from build123d import *

# Parameters (mm, degrees)
SKETCH1_W                  = 323
SKETCH1_H                  = 236
SKETCH1_W_2                = 286.7
SKETCH1_H_2                = 199.7
BOSS_EXTRUDE1_DEPTH        = 5
SKETCH2_W                  = 323
SKETCH2_H                  = 236
SKETCH2_W_2                = 297.2
SKETCH2_H_2                = 210.2
BOSS_EXTRUDE2_DEPTH        = 3.2
FILLET1_R                  = 10
FILLET2_R                  = 20
M4_TAPPED_HOLE1_AT_2_COUNT = 2
M4_TAPPED_HOLE1_AT_2_PITCH = 66.8
M4_TAPPED_HOLE1_AT_3_COUNT = 2
M4_TAPPED_HOLE1_AT_3_PITCH = 133.6
M4_TAPPED_HOLE1_AT_4_COUNT = 2
M4_TAPPED_HOLE1_AT_4_PITCH = 200.4
M4_TAPPED_HOLE1_AT_5_COUNT = 2
M4_TAPPED_HOLE1_AT_5_PITCH = 267.2
M4_TAPPED_HOLE2_AT_2_COUNT = 2
M4_TAPPED_HOLE2_AT_2_PITCH = 45.05
M4_TAPPED_HOLE2_AT_3_COUNT = 2
M4_TAPPED_HOLE2_AT_3_PITCH = 90.1
M4_TAPPED_HOLE2_AT_4_COUNT = 2
M4_TAPPED_HOLE2_AT_4_PITCH = 135.15
M4_TAPPED_HOLE2_AT_5_COUNT = 2
M4_TAPPED_HOLE2_AT_5_PITCH = 180.2
CHAMFER2_SIZE              = 3
SKETCH7_R                  = 3
CUT_EXTRUDE1_DEPTH         = 3.2
FILLET3_R                  = 10
CHAMFER3_SIZE              = 1
CUT_EXTRUDE2_DEPTH         = 2
CUT_EXTRUDE3_DEPTH         = 2


with BuildPart() as part:
    # Sketch1 → Boss-Extrude1 (new body)
    with BuildSketch(Plane(origin=(0, 0, 0), x_dir=(1, 0, 0), z_dir=(0, 1, 0))):
        Rectangle(SKETCH1_W, SKETCH1_H)
        Rectangle(SKETCH1_W_2, SKETCH1_H_2, mode=Mode.SUBTRACT)
    extrude(amount=BOSS_EXTRUDE1_DEPTH)

    # Sketch2 → Boss-Extrude2 (add)
    with BuildSketch(Plane.XZ):
        Rectangle(SKETCH2_W, SKETCH2_H)
        Rectangle(SKETCH2_W_2, SKETCH2_H_2, mode=Mode.SUBTRACT)
    extrude(amount=BOSS_EXTRUDE2_DEPTH)

    # Fillet1
    fillet1_edges = [part.edges().sort_by_distance(p)[0] for p in [
        (-143.35, 2.5, 99.85),
        (143.35, 2.5, 99.85),
        (143.35, 2.5, -99.85),
        (-143.35, 2.5, -99.85),
    ]]
    fillet(fillet1_edges, radius=FILLET1_R)

    # Fillet2
    fillet2_edges = [part.edges().sort_by_distance(p)[0] for p in [
        (-161.5, 0.9, 118),
        (-161.5, 0.9, -118),
        (161.5, 0.9, -118),
        (161.5, 0.9, 118),
    ]]
    fillet(fillet2_edges, radius=FILLET2_R)

    # Sketch4 → M4 Tapped Hole1 (revolve, cut)
    with BuildSketch(Plane(origin=(133.6, -3.2, -109), x_dir=(0, 0, -1), z_dir=(1, 0, 0))):
        Polygon((0, 0), (0, 6.991420021), (1.65, 6), (1.65, 0), align=None)
    m4_tapped_hole1 = revolve(axis=Axis((133.6, -9.55, -109), (0, 1, 0)), mode=Mode.SUBTRACT)

    # M4 Tapped Hole1 at 2: M4 Tapped Hole1 ×2
    with Locations(*[(-i * M4_TAPPED_HOLE1_AT_2_PITCH, 0, 0) for i in range(1, M4_TAPPED_HOLE1_AT_2_COUNT)]):
        add(m4_tapped_hole1, mode=Mode.SUBTRACT)

    # M4 Tapped Hole1 at 3: M4 Tapped Hole1 ×2
    with Locations(*[(-i * M4_TAPPED_HOLE1_AT_3_PITCH, 0, 0) for i in range(1, M4_TAPPED_HOLE1_AT_3_COUNT)]):
        add(m4_tapped_hole1, mode=Mode.SUBTRACT)

    # M4 Tapped Hole1 at 4: M4 Tapped Hole1 ×2
    with Locations(*[(-i * M4_TAPPED_HOLE1_AT_4_PITCH, 0, 0) for i in range(1, M4_TAPPED_HOLE1_AT_4_COUNT)]):
        add(m4_tapped_hole1, mode=Mode.SUBTRACT)

    # M4 Tapped Hole1 at 5: M4 Tapped Hole1 ×2
    with Locations(*[(-i * M4_TAPPED_HOLE1_AT_5_PITCH, 0, 0) for i in range(1, M4_TAPPED_HOLE1_AT_5_COUNT)]):
        add(m4_tapped_hole1, mode=Mode.SUBTRACT)

    # Mirror1: M4 Tapped Hole1 across plane
    add(m4_tapped_hole1.mirror(Plane.XY), mode=Mode.SUBTRACT)

    # Mirror1 copy 1 sketch → Mirror1 copy 1 (revolve, cut)
    with BuildSketch(Plane(origin=(66.8, -3.2, 109), x_dir=(0, 0, 1), z_dir=(1, 0, 0))):
        Polygon((0, 0), (0, -6.991420021), (1.65, -6), (1.65, 0), align=None)
    revolve(axis=Axis((66.8, -9.55, 109), (0, -1, 0)), mode=Mode.SUBTRACT)

    # Mirror1 copy 2 sketch → Mirror1 copy 2 (revolve, cut)
    with BuildSketch(Plane(origin=(0, -3.2, 109), x_dir=(0, 0, 1), z_dir=(1, 0, 0))):
        Polygon((0, 0), (0, -6.991420021), (1.65, -6), (1.65, 0), align=None)
    revolve(axis=Axis((0, -9.55, 109), (0, -1, 0)), mode=Mode.SUBTRACT)

    # Mirror1 copy 3 sketch → Mirror1 copy 3 (revolve, cut)
    with BuildSketch(Plane(origin=(-66.8, -3.2, 109), x_dir=(0, 0, 1), z_dir=(1, 0, 0))):
        Polygon((0, 0), (0, -6.991420021), (1.65, -6), (1.65, 0), align=None)
    revolve(axis=Axis((-66.8, -9.55, 109), (0, -1, 0)), mode=Mode.SUBTRACT)

    # Mirror1 copy 4 sketch → Mirror1 copy 4 (revolve, cut)
    with BuildSketch(Plane(origin=(-133.6, -3.2, 109), x_dir=(0, 0, 1), z_dir=(1, 0, 0))):
        Polygon((0, 0), (0, -6.991420021), (1.65, -6), (1.65, 0), align=None)
    revolve(axis=Axis((-133.6, -9.55, 109), (0, -1, 0)), mode=Mode.SUBTRACT)

    # Sketch6 → M4 Tapped Hole2 (revolve, cut)
    with BuildSketch(Plane(origin=(152.5, -3.2, -90.1), x_dir=(0, 0, -1), z_dir=(1, 0, 0))):
        Polygon((0, 0), (0, 7.091420021), (1.65, 6.1), (1.65, 0), align=None)
    m4_tapped_hole2 = revolve(axis=Axis((152.5, -9.55, -90.1), (0, 1, 0)), mode=Mode.SUBTRACT)

    # M4 Tapped Hole2 at 2: M4 Tapped Hole2 ×2
    with Locations(*[(0, 0, i * M4_TAPPED_HOLE2_AT_2_PITCH) for i in range(1, M4_TAPPED_HOLE2_AT_2_COUNT)]):
        add(m4_tapped_hole2, mode=Mode.SUBTRACT)

    # M4 Tapped Hole2 at 3: M4 Tapped Hole2 ×2
    with Locations(*[(0, 0, i * M4_TAPPED_HOLE2_AT_3_PITCH) for i in range(1, M4_TAPPED_HOLE2_AT_3_COUNT)]):
        add(m4_tapped_hole2, mode=Mode.SUBTRACT)

    # M4 Tapped Hole2 at 4: M4 Tapped Hole2 ×2
    with Locations(*[(0, 0, i * M4_TAPPED_HOLE2_AT_4_PITCH) for i in range(1, M4_TAPPED_HOLE2_AT_4_COUNT)]):
        add(m4_tapped_hole2, mode=Mode.SUBTRACT)

    # M4 Tapped Hole2 at 5: M4 Tapped Hole2 ×2
    with Locations(*[(0, 0, i * M4_TAPPED_HOLE2_AT_5_PITCH) for i in range(1, M4_TAPPED_HOLE2_AT_5_COUNT)]):
        add(m4_tapped_hole2, mode=Mode.SUBTRACT)

    # Mirror2: M4 Tapped Hole2 across plane
    add(m4_tapped_hole2.mirror(Plane(origin=(0, 0, 0), x_dir=(0, 0, 1), z_dir=(1, 0, 0))), mode=Mode.SUBTRACT)

    # Mirror2 copy 1 sketch → Mirror2 copy 1 (revolve, cut)
    with BuildSketch(Plane(origin=(-152.5, -3.2, -45.05), x_dir=(0, 0, -1), z_dir=(-1, 0, 0))):
        Polygon((0, 0), (0, -7.091420021), (1.65, -6.1), (1.65, 0), align=None)
    revolve(axis=Axis((-152.5, -9.55, -45.05), (0, -1, 0)), mode=Mode.SUBTRACT)

    # Mirror2 copy 2 sketch → Mirror2 copy 2 (revolve, cut)
    with BuildSketch(Plane(origin=(-152.5, -3.2, 0), x_dir=(0, 0, -1), z_dir=(-1, 0, 0))):
        Polygon((0, 0), (0, -7.091420021), (1.65, -6.1), (1.65, 0), align=None)
    revolve(axis=Axis((-152.5, -9.55, 0), (0, -1, 0)), mode=Mode.SUBTRACT)

    # Mirror2 copy 3 sketch → Mirror2 copy 3 (revolve, cut)
    with BuildSketch(Plane(origin=(-152.5, -3.2, 45.05), x_dir=(0, 0, -1), z_dir=(-1, 0, 0))):
        Polygon((0, 0), (0, -7.091420021), (1.65, -6.1), (1.65, 0), align=None)
    revolve(axis=Axis((-152.5, -9.55, 45.05), (0, -1, 0)), mode=Mode.SUBTRACT)

    # Mirror2 copy 4 sketch → Mirror2 copy 4 (revolve, cut)
    with BuildSketch(Plane(origin=(-152.5, -3.2, 90.1), x_dir=(0, 0, -1), z_dir=(-1, 0, 0))):
        Polygon((0, 0), (0, -7.091420021), (1.65, -6.1), (1.65, 0), align=None)
    revolve(axis=Axis((-152.5, -9.55, 90.1), (0, -1, 0)), mode=Mode.SUBTRACT)

    # Chamfer2
    chamfer2_edges = [part.edges().sort_by_distance(p)[0] for p in [
        (0, 5, 118),
        (-161.5, 5, 0),
        (161.5, 5, 0),
        (0, 5, -118),
        (-155.642135624, 5, -112.142135624),
        (155.642135624, 5, 112.142135624),
        (155.642135624, 5, -112.142135624),
        (-155.642135624, 5, 112.142135624),
    ]]
    chamfer(chamfer2_edges, length=CHAMFER2_SIZE)

    # Sketch7 → Cut-Extrude1 (cut)
    with BuildSketch(Plane.XZ.offset(3.2)):
        with Locations((147.3, -103.8)):
            Circle(SKETCH7_R)
        with Locations((-147.3, -103.8)):
            Circle(SKETCH7_R)
        with Locations((-147.3, 103.8)):
            Circle(SKETCH7_R)
        with Locations((147.3, 103.8)):
            Circle(SKETCH7_R)
    extrude(amount=-CUT_EXTRUDE1_DEPTH, mode=Mode.SUBTRACT)

    # Fillet3
    fillet3_edges = [part.edges().sort_by_distance(p)[0] for p in [
        (144.596298833, -1.6, -105.1),
        (-144.596298833, -1.6, -105.1),
        (-148.6, -1.6, 101.096298833),
        (144.596298833, -1.6, 105.1),
        (148.6, -1.6, 101.096298833),
        (-144.596298833, -1.6, 105.1),
        (-148.6, -1.6, -101.096298833),
        (148.6, -1.6, -101.096298833),
    ]]
    fillet(fillet3_edges, radius=FILLET3_R)

    # Chamfer3
    chamfer3_edges = [part.edges().sort_by_distance(p)[0] for p in [
        (0, 5, 99.85),
        (143.35, 5, 0),
        (0, 5, -99.85),
        (-143.35, 5, 0),
        (140.421067812, 5, 96.921067812),
        (140.421067812, 5, -96.921067812),
        (-140.421067812, 5, 96.921067812),
        (-140.421067812, 5, -96.921067812),
    ]]
    chamfer(chamfer3_edges, length=CHAMFER3_SIZE)

    # Sketch8 → Cut-Extrude2 (cut)
    with BuildSketch(Plane.XZ):
        with BuildLine():
            Line((148.6, -89.85), (148.6, 89.85))
            ThreePointArc((148.6, 89.85), (144.133378413, 100.633378413), (133.35, 105.1))
            Line((133.35, 105.1), (-133.35, 105.1))
            ThreePointArc((-133.35, 105.1), (-144.133378413, 100.633378413), (-148.6, 89.85))
            Line((-148.6, 89.85), (-148.6, -89.85))
            ThreePointArc((-148.6, -89.85), (-144.133378413, -100.633378413), (-133.35, -105.1))
            Line((-133.35, -105.1), (133.35, -105.1))
            ThreePointArc((133.35, -105.1), (144.133378413, -100.633378413), (148.6, -89.85))
        make_face()
        with BuildLine():
            Line((133.35, 101.85), (-133.35, 101.85))
            ThreePointArc((-133.35, 101.85), (-141.835281374, 98.335281374), (-145.35, 89.85))
            Line((-145.35, 89.85), (-145.35, -89.85))
            ThreePointArc((-145.35, -89.85), (-141.835281374, -98.335281374), (-133.35, -101.85))
            Line((-133.35, -101.85), (133.35, -101.85))
            ThreePointArc((133.35, -101.85), (141.835281374, -98.335281374), (145.35, -89.85))
            Line((145.35, -89.85), (145.35, 89.85))
            ThreePointArc((145.35, 89.85), (141.835281374, 98.335281374), (133.35, 101.85))
        make_face(mode=Mode.SUBTRACT)
    extrude(amount=-CUT_EXTRUDE2_DEPTH, mode=Mode.SUBTRACT)

    # Sketch9 → Cut-Extrude3 (cut)
    with BuildSketch(Plane.XZ.offset(3.2)):
        with BuildLine():
            Line((141.5, 116), (-141.5, 116))
            ThreePointArc((-141.5, 116), (-154.227922061, 110.727922061), (-159.5, 98))
            Line((-159.5, 98), (-159.5, -98))
            ThreePointArc((-159.5, -98), (-154.227922061, -110.727922061), (-141.5, -116))
            Line((-141.5, -116), (141.5, -116))
            ThreePointArc((141.5, -116), (154.227922061, -110.727922061), (159.5, -98))
            Line((159.5, -98), (159.5, 98))
            ThreePointArc((159.5, 98), (154.227922061, 110.727922061), (141.5, 116))
        make_face()
        with BuildLine():
            Line((156.25, -98), (156.25, 98))
            ThreePointArc((156.25, 98), (151.929825023, 108.429825023), (141.5, 112.75))
            Line((141.5, 112.75), (-141.5, 112.75))
            ThreePointArc((-141.5, 112.75), (-151.929825023, 108.429825023), (-156.25, 98))
            Line((-156.25, 98), (-156.25, -98))
            ThreePointArc((-156.25, -98), (-151.929825023, -108.429825023), (-141.5, -112.75))
            Line((-141.5, -112.75), (141.5, -112.75))
            ThreePointArc((141.5, -112.75), (151.929825023, -108.429825023), (156.25, -98))
        make_face(mode=Mode.SUBTRACT)
    extrude(amount=-CUT_EXTRUDE3_DEPTH, mode=Mode.SUBTRACT)


solid = part.part
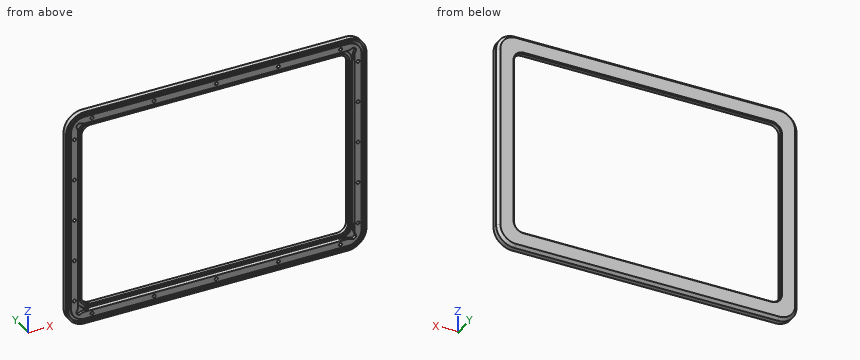
Source: CAD feature listing. Evaluate the final solid. Frame: model axes, mm. Give positions to 0.01 mm unless a question says otherwise; leave off trailing zeros. Order: outer loops, then holes, each group sorted by start corner. A loop starts at its lowest first (then second) coordinate and runs counter-clockwise, first axis right, second up. Notation, with made-up numbers: (72.5, 7) -> (80.5, 7) arc R23 ccw to (80.5, 44) -> close; hole circle Ø9 at (62, 19). An arc over 180 degrees is marked (long way). Write item = value, one per line.
Item 1: Section query B-B (z = -54). Output: boundary loops of the cut face in (x, y), then the cut area to 3 significant figures.
Check result:
outline = (-161.5, -3.2) -> (-159.5, -3.2) -> (-159.5, -1.2) -> (-156.25, -1.2) -> (-156.25, -3.2) -> (-148.6, -3.2) -> (-148.6, 2) -> (-145.35, 2) -> (-145.35, 0) -> (-143.35, 0) -> (-143.35, 4) -> (-144.35, 5) -> (-158.5, 5) -> (-161.5, 2) -> close; (143.35, 0) -> (145.35, 0) -> (145.35, 2) -> (148.6, 2) -> (148.6, -3.2) -> (156.25, -3.2) -> (156.25, -1.2) -> (159.5, -1.2) -> (159.5, -3.2) -> (161.5, -3.2) -> (161.5, 2) -> (158.5, 5) -> (144.35, 5) -> (143.35, 4) -> close
area = 228 mm²
Item 2: Ray query, probe 1 along X at (y, z) = (0.75, 60); probe 2 along X at (y, z) = (-0.25, 90.1); probe 3 along Z at (x, y) = (-54.5, -1.5). Return the intervals inside material, ascending.
Check result:
probe_1 = -161.5 to -148.6, -145.35 to -143.35, 143.35 to 145.35, 148.6 to 161.5
probe_2 = -161.5 to -154.15, -150.85 to -148.6, 148.6 to 150.85, 154.15 to 161.5
probe_3 = -118 to -116, -112.75 to -105.1, 105.1 to 112.75, 116 to 118
Item 3: Contact query for flat-ended pins moving along their axis: pin 1 (5 mm diameter, centred on x = -139, z = -101.5, fed in from -Y); pin 2 (2 mm diameter, centred on x = 66.8, z = 109, fed in from -Y); pin 3 (2 mm diameter, centred on x = -152.5, z = 90.1, fed in from -Y). Output: stop coordinate, or through.
Check result:
pin_1 = 0
pin_2 = 3.19
pin_3 = 3.29
Item 4: Section query A-A (x = 54.5). Output: boundary loops of the cut face in (y, z), then the cut area to 3 significant figures.
Check result:
outline = (-3.2, -118) -> (2, -118) -> (5, -115) -> (5, -100.85) -> (4, -99.85) -> (0, -99.85) -> (0, -101.85) -> (2, -101.85) -> (2, -105.1) -> (-3.2, -105.1) -> (-3.2, -112.75) -> (-1.2, -112.75) -> (-1.2, -116) -> (-3.2, -116) -> close; (-3.2, 105.1) -> (2, 105.1) -> (2, 101.85) -> (0, 101.85) -> (0, 99.85) -> (4, 99.85) -> (5, 100.85) -> (5, 115) -> (2, 118) -> (-3.2, 118) -> (-3.2, 116) -> (-1.2, 116) -> (-1.2, 112.75) -> (-3.2, 112.75) -> close
area = 228 mm²
